The figure shows three views and two pictorial views of one solid part (mm, origin at its lowest corner). Answer the questions. A direction names the side the tool comes from. Give positions to 0.01 mm unless a question says otherwise; leave off trailing zeros. Write each loop counter-clockwise with the first axis right and the second up, starting at its lowest first coordinate (ties: lowest second). Pieces come first, ordered by that corner, then holes. Notation, with made-up numbers: (1.5, 49.5) -> (33.5, 49.5) arc R36 ccw to (33.5, 87.5) -> close; hole circle Ø8 at (-19, 15). An arc over 180 degrees is marked (long way). Write each question's results on one line, items separated by ' | '. Start each with the question number.
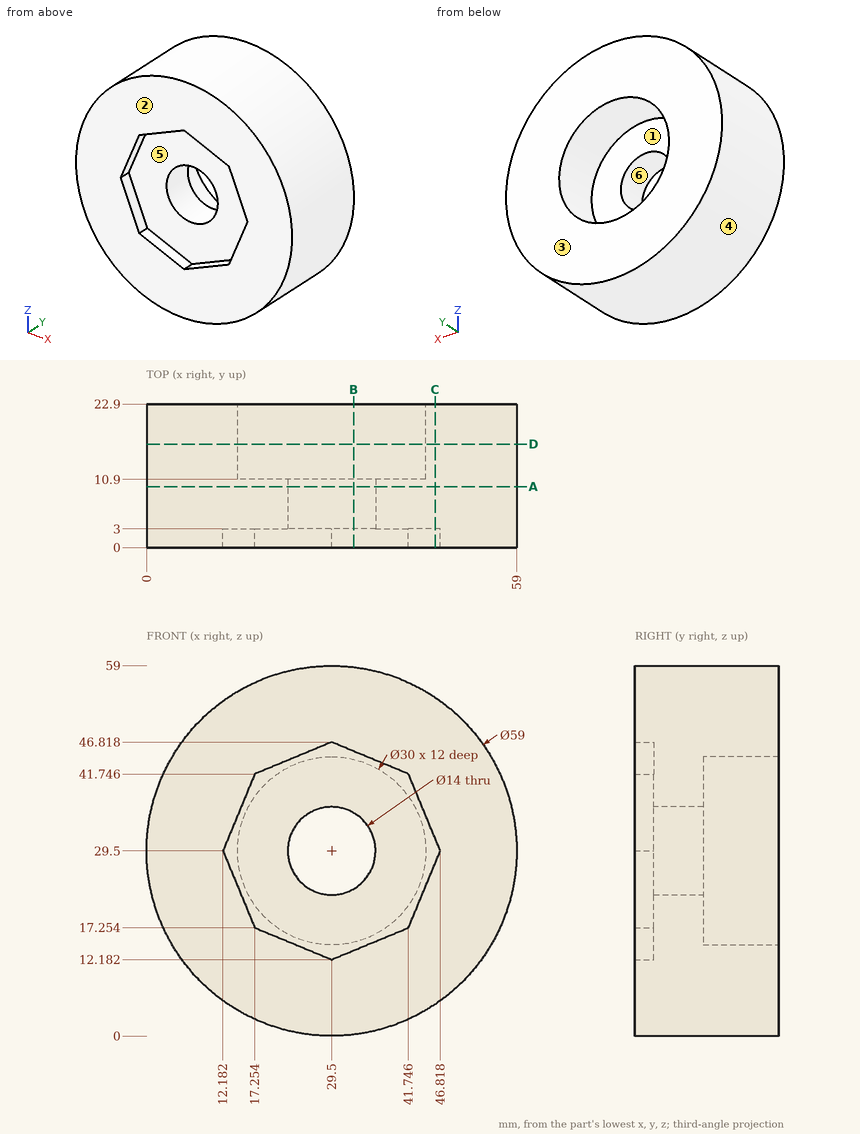
1. Section C-C (x = 46) is taken. Write down the section's boundary in (y, z) (1 decimal), then the cut area to 3 significant figures.
2. Section A-A (y = 9.75) is taken. Write down the section's boundary in (x, z).
3. The mould has two halves that part along Z. Classify the marked faces 3, 4, 5 and 6: pulls with the +Z half, pulls with the -Z half, needs draft (parallel to the pull), parting line crosses it, or undercut.
4. Each of these flat-tipped pins is pushed along its axis until it touches: pin 1 Ø12 at (y, z) = (20, 51.5) entering from -X; pin 2 Ø10 at (y, z) = (12.5, 30.5) entering from +X; pin 3 Ø1.5 at (x, y) = (39.5, 12) entering from +Z. Where does it stop, or does it pass through?
5. A tool of negligible diameter and unlimited length cuts with its end or side. For the marked faces 1 and 2, from which of +Z, -Z, +X, -X, +Y, -Y can it reach the whole face along a straight path? Write none if from no direction.
6. Section B-B (x = 33) is taken. Write down the section's boundary in (y, z).
7. Consider probe 1 along X at (y, z) = (5.75, 29.5); probe 2 along X at (y, z) = (18, 29.5); probe 3 along Z at (x, y) = (27.5, 16). Determine where each line is inside the solid, lowest interval first. Write a range as [from, to].
8. Section D-D (y = 16.5) is taken. Write down the section's boundary in (x, z).
Results:
1) outline: (0, 5) -> (22.9, 5) -> (22.9, 54) -> (0, 54) -> (0, 31.5) -> (3, 31.5) -> (3, 27.5) -> (0, 27.5) -> close | area: 1,110 mm²
2) outline: circle Ø59 at (29.5, 29.5); hole circle Ø14 at (29.5, 29.5)
3) face 3: needs draft | face 4: parting line crosses it | face 5: undercut | face 6: undercut
4) pin 1: stops at x = 4.72 | pin 2: stops at x = 59 | pin 3: stops at z = 57.51
5) face 1: +Y | face 2: +Z, -Z, +X, -X, -Y
6) outline: (0, 0.21) -> (22.9, 0.21) -> (22.9, 14.91) -> (10.9, 14.91) -> (10.9, 23.44) -> (3, 23.44) -> (3, 13.63) -> (0, 13.63) -> close; (0, 45.37) -> (3, 45.37) -> (3, 35.56) -> (10.9, 35.56) -> (10.9, 44.09) -> (22.9, 44.09) -> (22.9, 58.79) -> (0, 58.79) -> close
7) probe 1: x = [0, 22.5], [36.5, 59] | probe 2: x = [0, 14.5], [44.5, 59] | probe 3: z = [0.07, 14.63], [44.37, 58.93]
8) outline: circle Ø59 at (29.5, 29.5); hole circle Ø30 at (29.5, 29.5)
